Autodesk Inventor part; units mm, degrees
ref_plane "YZ Plane" through (0, 0, 0) normal (1, 0, 0) x (0, 1, 0)
ref_plane "XZ Plane" through (0, 0, 0) normal (0, 1, 0) x (-1, 0, 0)
ref_plane "XY Plane" through (0, 0, 0) normal (0, 0, 1) x (1, 0, 0)
sketch "Sketch1" plane through (0, 0, 0) normal (0, 0, 1) x (1, 0, 0)
  circle A0 centre (0, 0) radius 3.175
  circle A1 centre (0, 0) radius 1.7272
  line L0 (0.5499, 0.9525) -> (1.0999, 0)
  line L1 (1.0999, 0) -> (0.5499, -0.9525)
  line L2 (0.5499, -0.9525) -> (-0.5499, -0.9525)
  line L3 (-0.5499, -0.9525) -> (-1.0999, 0)
  line L4 (-1.0999, 0) -> (-0.5499, 0.9525)
  line L5 (-0.5499, 0.9525) -> (0.5499, 0.9525)
  dimension "d0" = 3.4544
  dimension "d1" = 6.35
  dimension "d2" = 1.905
extrude "Extrusion1" add sketch "Sketch1" against normal blind 12.7 contours A1 | L0 L1 L2 L3 L4 L5
extrude "Extrusion2" add sketch "Sketch1" along normal blind 1.5875 contours A0 | A1
extrude "Extrusion3" add sketch "Sketch1" along normal blind 0.7937 contours L0 L1 L2 L3 L4 L5
thread "Thread1"
chamfer "Chamfer1" distance 0.3969 angle 45 1 edges at (-1.7272, 0, -12.7)
fillet "Fillet1" radius 1.5875 1 edges at (-3.175, 0, 1.5875)
properties part number "6 32 bolt 0.5''"
Build history of the part. All positions in model axes, mm. Round coordinates to 2 decimals unless told otherwise and drop trailing zeros. Loops run counter-clockwise (first coordinate to the right, second up) from the corner with the lowest first, then second, coordinate; pieces in that order, holes last. Notation, with made-up numbers: (-14.75, -8.75) -> (0.25, -8.75) arc R29 cw to (0.25, 16.25) -> close; hole circle Ø1 at (5, 51.5). An arc over 180 degrees is marked (long way). Answer in a Markdown table with one row per item.
Item 1: Saw through at B-B (z = -4.5). Write the cut outline in (x, y), and give its area (3 significant figures).
Answers below:
| item | result |
|---|---|
| outline | circle Ø3.45 at (0, 0) |
| area | 9.37 mm² |
Item 2: Drill centre lines: L1, parallel to Y at x = 0, z = -1; L2, parallel to Z at x = -0.25, y = 0.75; L3, parallel to X at y = -0.5, z = -8. Where is each one in solid material? Low to high. Write a range as [from, to].
Answers below:
| item | result |
|---|---|
| L1 | y = [-1.73, 1.73] |
| L2 | z = [-12.7, 0.79] |
| L3 | x = [-1.65, 1.65] |
Item 3: Pin check, flat tips, straight feed: pin 1 (1.5 mm diameter, centred on x = -1.5, z = -4.5, fed in from -Y); pin 2 (0.6 mm diameter, centred on x = -0.5, z = 1.5, fed in from -Y); pin 3 (2 mm diameter, centred on x = -0.5, z = -9, fed in from -Y). Stop position of each tip, or through.
Answers below:
| item | result |
|---|---|
| pin 1 | stops at y = -1.56 |
| pin 2 | stops at y = -2.58 |
| pin 3 | stops at y = -1.73 |
Item 4: Mould opens along Y. For faces 1 (the flat face through (0, 0, 0.794)), 2 (the cylindrical face through (-0.225, 1.713, -6.065)), 3 (the flat face through (1.4, -1.4, 0)) say: +Y half, -Y half, draft (parallel to the pull), parting line (faces both ways), or undercut.
Answers below:
| item | result |
|---|---|
| face 1 | undercut |
| face 2 | parting line |
| face 3 | draft |
